Verification items for the finished model (mm, model axes). Face numbers are marked on the shaded views. A direction names the side the tool comes from. Round coordinates to 2 decimals unless told otherwise and drop trailing zeros. Write each loop counter-clockwise with the first axis right and the second up, starting at its lowest first coordinate (ties: lowest second). Pieces come first, ordered by that corner, then holes. Notation, with made-up numbers: M -8.5,83.25 L 25.5,83.25 A5 ccw 25.5,92.25 Z; hole C 1,-18.75 d2. An arc over 180 degrees is marked long. Answer in a Markdown table with one row per item. Add a question column.
1. Sectioned sample at B-B on x = 0. Record the cut outline in (y, z), plus the area to 3 significant figures.
2. Sectioned sample at C-C on y = -15. Record the cut outline in (x, z).
3. Draft check along Z on the marked faces 1, 2, 3 and 4. Enter one of: pulls with the +Z half, pulls with the -Z half, needs draft (parallel to the pull), parting line crosses it, or undercut.
4. Sectioned sample at A-A on z = 0. Record the cut outline in (x, y), plus the area to 3 significant figures.
5. Material ranges on probe 1 along Z at (x, y) = (37, 7); probe 2 along X at (y, z) = (5.5, 11); probe 3 along X at (y, z) = (4.5, 8), recorded low to high.
6. Go/stop test with flat-tipped pins: pin 1 Ø6 at (x, y) = (24, -5.5) entering from +Z; pin 2 Ø13 at (x, z) = (-37, 11) entering from -Y; pin 3 Ø0.8 at (x, z) = (9.5, -1) entering from -Y; pin 4 Ø17 at (x, z) = (1.5, -13) entering from +Y. Record where each tip stops, or that it passes through.
7. Set-up check for the marked faces 5, 6, 7 and 8: record each of +Z, -Z, +X, -X, +Y, -Y from which the full face is reachable in a straight line by a thin tool's end or side.
8. Sectioned sample at D-D on y = -3.5. Record the cut outline in (x, z) (3 decimals).
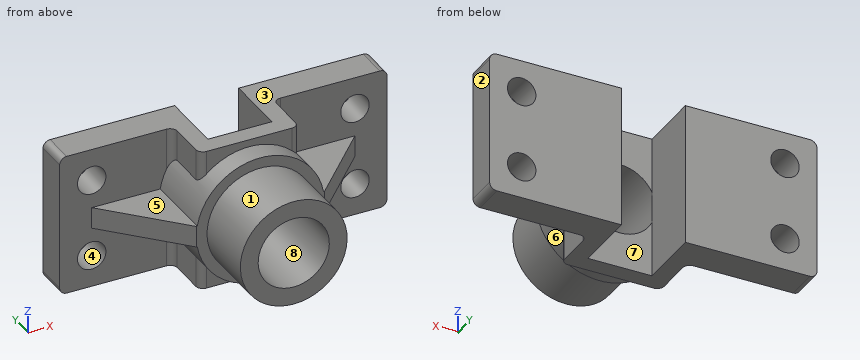
```python
from build123d import *

# Parameters (mm, degrees)
SKETCH1_W           = 92
SKETCH1_H           = 40
SKETCH1_R           = 4
BOSS_EXTRUDE2_DEPTH = 9
SKETCH3_R           = 18
SKETCH3_R_2         = 10
BOSS_EXTRUDE3_DEPTH = 20
SKETCH4_R           = 15
SKETCH4_R_2         = 10
BOSS_EXTRUDE4_DEPTH = 18
CUT_EXTRUDE1_REACH  = 73.833
SKETCH8_W           = 18
SKETCH8_H           = 18
CUT_EXTRUDE2_REACH  = 73.833
SKETCH9_W           = 28
SKETCH9_H           = 14
BOSS_EXTRUDE5_DEPTH = 40
BOSS_EXTRUDE9_DEPTH = 3
CUT_EXTRUDE5_REACH  = 73.833
SKETCH8_3_W         = 18
SKETCH8_3_H         = 18
CUT_EXTRUDE6_START  = -6
CUT_EXTRUDE6_DEPTH  = 6
CUT_EXTRUDE7_START  = -5
SKETCH19_R          = 10
CUT_EXTRUDE7_DEPTH  = 5
FILLET1_R           = 2
FILLET2_R           = 2


with BuildPart() as part:
    # Sketch1 → Boss-Extrude2 (new body)
    with BuildSketch(Plane(origin=(0, 0, 0), x_dir=(1, 0, 0), z_dir=(0, 1, 0))):
        Rectangle(SKETCH1_W, SKETCH1_H)
        with Locations(Location((-37, 11, 0), (0, 0, 270))):
            Circle(SKETCH1_R, mode=Mode.SUBTRACT)
        with Locations(Location((-37, -11, 0), (0, 0, 270))):
            Circle(SKETCH1_R, mode=Mode.SUBTRACT)
        with Locations(Location((37, -11, 0), (0, 0, 90))):
            Circle(SKETCH1_R, mode=Mode.SUBTRACT)
        with Locations(Location((37, 11, 0), (0, 0, 90))):
            Circle(SKETCH1_R, mode=Mode.SUBTRACT)
    extrude(amount=BOSS_EXTRUDE2_DEPTH)

    # Sketch3 → Boss-Extrude3 (add)
    with BuildSketch(Plane.XZ):
        with Locations(Location((0, 0, 0), (0, 0, 270))):
            Circle(SKETCH3_R)
        with Locations(Location((0, 0, 0), (0, 0, 270))):
            Circle(SKETCH3_R_2, mode=Mode.SUBTRACT)
    extrude(amount=BOSS_EXTRUDE3_DEPTH)

    # Sketch4 → Boss-Extrude4 (add)
    with BuildSketch(Plane.XZ.offset(20)):
        with Locations(Location((0, 0, 0), (0, 0, 270))):
            Circle(SKETCH4_R)
        with Locations(Location((0, 0, 0), (0, 0, 270))):
            Circle(SKETCH4_R_2, mode=Mode.SUBTRACT)
    extrude(amount=BOSS_EXTRUDE4_DEPTH)

    # Sketch8 → Cut-Extrude1 (cut, up to next)
    with BuildSketch(Plane.XY.offset(20), mode=Mode.PRIVATE) as cut_extrude1_sk1:
        Rectangle(SKETCH8_W, SKETCH8_H)
    cut_extrude1_tool1 = extrude(cut_extrude1_sk1.sketch, amount=-CUT_EXTRUDE1_REACH, mode=Mode.PRIVATE) & part.part
    add(cut_extrude1_tool1.solids().sort_by_distance((0, 0, 20))[0], mode=Mode.SUBTRACT)

    # Sketch9 → Cut-Extrude2 (cut, up to next)
    with BuildSketch(Plane.XY.offset(20), mode=Mode.PRIVATE) as cut_extrude2_sk1:
        with Locations((0, -7)):
            Rectangle(SKETCH9_W, SKETCH9_H)
    cut_extrude2_tool1 = extrude(cut_extrude2_sk1.sketch, amount=-CUT_EXTRUDE2_REACH, mode=Mode.PRIVATE) & part.part
    add(cut_extrude2_tool1.solids().sort_by_distance((0, -7, 20))[0], mode=Mode.SUBTRACT)

    # Sketch10 → Boss-Extrude5 (add)
    with BuildSketch(Plane.XY.offset(20)):
        Polygon((9, 0), (9, -9), (-8.881269958, -9), (-9, 0), (-14, 0), (-14, -14), (14, -14), (14, 0), align=None)
    extrude(amount=-BOSS_EXTRUDE5_DEPTH)

    # Sketch13 → Boss-Extrude9 (add, symmetric)
    with BuildSketch(Plane.XY):
        Polygon((-18, -20), (-37, 0), (-18, 0), (-9, 0), (9, 0), (18, 0), (37, 0), (18, -20), align=None)
    extrude(amount=BOSS_EXTRUDE9_DEPTH, both=True)

    # Sketch8<3> → Cut-Extrude5 (cut, up to next)
    with BuildSketch(Plane.XY.offset(20), mode=Mode.PRIVATE) as cut_extrude5_sk1:
        Rectangle(SKETCH8_3_W, SKETCH8_3_H)
    cut_extrude5_tool1 = extrude(cut_extrude5_sk1.sketch, amount=-CUT_EXTRUDE5_REACH, mode=Mode.PRIVATE) & part.part
    add(cut_extrude5_tool1.solids().sort_by_distance((0, 0, 20))[0], mode=Mode.SUBTRACT)

    # Sketch18 → Cut-Extrude6 (cut)
    with BuildSketch(Plane.XZ.offset(20).offset(CUT_EXTRUDE6_START)):
        with BuildLine():
            Line((9.539392014, 3), (-9.539392014, 3))
            ThreePointArc((-9.539392014, 3), (-10, 0), (-9.539392014, -3))
            Line((-9.539392014, -3), (9.539392014, -3))
            ThreePointArc((9.539392014, -3), (10, 0), (9.539392014, 3))
        make_face()
    extrude(amount=CUT_EXTRUDE6_DEPTH, mode=Mode.SUBTRACT)

    # Sketch19 → Cut-Extrude7 (cut)
    with BuildSketch(Plane.XZ.offset(14).offset(CUT_EXTRUDE7_START)):
        with Locations(Location((0, 0, 0), (0, 0, 25.841932763))):
            Circle(SKETCH19_R)
    extrude(amount=CUT_EXTRUDE7_DEPTH, mode=Mode.SUBTRACT)

    # Fillet1
    fillet1_edges = [part.edges().sort_by_distance(p)[0] for p in [
        (46, 4.5, 20),
        (-46, 4.5, 20),
        (-46, 4.5, -20),
        (46, 4.5, -20),
    ]]
    fillet(fillet1_edges, radius=FILLET1_R)

    # Fillet2
    fillet2_edges = [part.edges().sort_by_distance(p)[0] for p in [
        (14, -14, 15.656854249),
        (14, -14, -15.656854249),
        (14, 0, -15.656854249),
        (14, 0, 15.656854249),
        (-14, -14, 15.656854249),
        (-14, -14, -15.656854249),
        (-14, 0, -15.656854249),
        (-14, 0, 15.656854249),
    ]]
    fillet(fillet2_edges, radius=FILLET2_R)


solid = part.part
```
Geometry check:
| question | item | result |
|---|---|---|
| 1 | outline | M -38,-15 L -20,-15 L -20,-18 L -14,-18 L -14,-20 L -9,-20 L -9,-10 L -38,-10 Z; M -38,10 L -9,10 L -9,20 L -14,20 L -14,18 L -20,18 L -20,15 L -38,15 Z |
| 1 | area | 376 mm2 |
| 2 | outline | M -22.75,-3 L -17.75,-3 A18 ccw 17.75,-3 L 22.75,-3 L 22.75,3 L 17.75,3 A18 ccw -17.75,3 L -22.75,3 Z; hole C 0,0 d20 |
| 3 | face 1 | parting line crosses it |
| 3 | face 2 | needs draft |
| 3 | face 3 | pulls with the +Z half |
| 3 | face 4 | undercut |
| 4 | outline | M -46,0 L -37,0 L -18,-20 L -15,-20 L -15,-38 L -10,-38 L -10,-9 L -9,-9 L -9,9 L -46,9 Z; M 9,-9 L 10,-9 L 10,-38 L 15,-38 L 15,-20 L 18,-20 L 37,0 L 46,0 L 46,9 L 9,9 Z |
| 4 | area | 1,560 mm2 |
| 5 | probe 1 | z = -20 to -15, -7 to 7, 15 to 20 |
| 5 | probe 2 | x = -46 to -41, -33 to -9, 9 to 33, 41 to 46 |
| 5 | probe 3 | x = -46 to -39.65, -34.35 to -9, 9 to 34.35, 39.65 to 46 |
| 6 | pin 1 | stops at z = 3 |
| 6 | pin 2 | stops at y = 0 |
| 6 | pin 3 | stops at y = -9 |
| 6 | pin 4 | stops at y = 9 |
| 7 | face 5 | +Z, -X, -Y |
| 7 | face 6 | -Z, -Y |
| 7 | face 7 | +Z, -Z, +Y |
| 7 | face 8 | -Y |
| 8 | outline | M -33.675,-3 L -17.748,-3 A18 ccw -14,-11.314 L -14,-20 L -9,-20 L -9,20 L -14,20 L -14,11.314 A18 ccw -17.748,3 L -33.675,3 Z; M 9,-20 L 14,-20 L 14,-11.314 A18 ccw 17.748,-3 L 33.675,-3 L 33.675,3 L 17.748,3 A18 ccw 14,11.314 L 14,20 L 9,20 Z |
